from build123d import *

# Parameters (mm, degrees)
SKETCH1_W            = 34.7
SKETCH1_H            = 30
BOSS_EXTRUDE1_DEPTH  = 37.282
SKETCH4_R            = 5.715
CUT_EXTRUDE1_DEPTH   = 31
SKETCH8_W            = 3.81
SKETCH8_H            = 50.8
BOSS_EXTRUDE6_DEPTH  = 45.72
BOSS_EXTRUDE7_DEPTH  = 41.000001
CUT_EXTRUDE2_REACH   = 82.42
SKETCH10_R           = 1.905
SKETCH11_W           = 12.7
SKETCH11_H           = 44.810000611
BOSS_EXTRUDE8_DEPTH  = 12.7
SKETCH12_W           = 12.7
SKETCH12_H           = 44.810000611
BOSS_EXTRUDE9_DEPTH  = 12.7
SKETCH13_R           = 4.25
CUT_EXTRUDE3_DEPTH   = 6.35
SKETCH17_W           = 3.43592392
SKETCH17_H           = 45.72
BOSS_EXTRUDE12_DEPTH = 33.472
SKETCH16_W           = 2.5
SKETCH16_H           = 37.282
BOSS_EXTRUDE11_DEPTH = 9.076061
SKETCH21_W           = 17.974491303
SKETCH21_H           = 23.94
BOSS_EXTRUDE13_DEPTH = 16
SKETCH22_W           = 13.379509134
SKETCH22_H           = 6.922502695
CUT_EXTRUDE4_DEPTH   = 45.810000611
SKETCH23_W           = 13.335762063
SKETCH23_H           = 11.735762062
CUT_EXTRUDE5_DEPTH   = 21.47692
SKETCH24_W           = 22.672584076
SKETCH24_H           = 14.765845737
BOSS_EXTRUDE14_DEPTH = 15
SKETCH25_W           = 12.9
SKETCH25_H           = 11.3
CUT_EXTRUDE6_DEPTH   = 22.672584
SKETCH5_R            = 1.375
CUT_EXTRUDE7_DEPTH   = 10
SKETCH6_R            = 1.27
CUT_EXTRUDE8_DEPTH   = 53.282
SKETCH27_W           = 17.974491303
SKETCH27_H           = 14.491353785
BOSS_EXTRUDE15_DEPTH = 2


with BuildPart() as part:
    # Sketch1 → Boss-Extrude1 (new body)
    with BuildSketch(Plane(origin=(0, 0, -264.675), x_dir=(-1, 0, 0), z_dir=(0, 0, -1))):
        with Locations((-46.026450848, -396.896376681)):
            Rectangle(SKETCH1_W, SKETCH1_H)
    extrude(amount=BOSS_EXTRUDE1_DEPTH)

    # Sketch4 → Cut-Extrude1 (cut, through all)
    with BuildSketch(Plane(origin=(0, -381.896376681, 0), x_dir=(1, 0, 0), z_dir=(0, 1, 0))):
        with Locations((46.026450848, 283.749893694)):
            Circle(SKETCH4_R)
    extrude(amount=-CUT_EXTRUDE1_DEPTH, mode=Mode.SUBTRACT)

    # Sketch8 → Boss-Extrude6 (add)
    with BuildSketch(Plane(origin=(63.376450848, 0, 0), x_dir=(0, 0, -1), z_dir=(1, 0, 0))):
        with Locations((266.58, -395.572437442)):
            Rectangle(SKETCH8_W, SKETCH8_H)
    extrude(amount=BOSS_EXTRUDE6_DEPTH)

    # Sketch9 → Boss-Extrude7 (add)
    with BuildSketch(Plane(origin=(0, 0, -268.485), x_dir=(-1, 0, 0), z_dir=(0, 0, -1))):
        Polygon((-109.096450848, -370.172437442), (-63.376450848, -370.172437442), (-63.376450848, -372.712437442), (-106.556450848, -372.712437442), (-106.556450848, -384.142437442), (-109.096450848, -384.142437442), (-109.096450848, -372.712437442), align=None)
        Polygon((-109.096450848, -420.972437442), (-63.376450848, -420.972437442), (-63.376450848, -418.432437442), (-106.556450848, -418.432437442), (-106.556450848, -407.002437442), (-109.096450848, -407.002437442), (-109.096450848, -418.432437442), align=None)
    extrude(amount=BOSS_EXTRUDE7_DEPTH)

    # Sketch10 → Cut-Extrude2 (cut, up to next)
    with BuildSketch(Plane(origin=(109.096450848, 0, 0), x_dir=(0, 0, -1), z_dir=(1, 0, 0)), mode=Mode.PRIVATE) as cut_extrude2_sk1:
        with Locations((304.963451053, -379.773986799)):
            Circle(SKETCH10_R)
    cut_extrude2_tool1 = extrude(cut_extrude2_sk1.sketch, amount=-CUT_EXTRUDE2_REACH, mode=Mode.PRIVATE) & part.part
    add(cut_extrude2_tool1.solids().sort_by_distance((109.096451, -379.773987, -304.963451))[0], mode=Mode.SUBTRACT)
    # Sketch10 → Cut-Extrude2 (cut, up to next)
    with BuildSketch(Plane(origin=(109.096450848, 0, 0), x_dir=(0, 0, -1), z_dir=(1, 0, 0)), mode=Mode.PRIVATE) as cut_extrude2_sk2:
        with Locations((304.941901697, -411.752437852)):
            Circle(SKETCH10_R)
    cut_extrude2_tool2 = extrude(cut_extrude2_sk2.sketch, amount=-CUT_EXTRUDE2_REACH, mode=Mode.PRIVATE) & part.part
    add(cut_extrude2_tool2.solids().sort_by_distance((109.096451, -411.752438, -304.941902))[0], mode=Mode.SUBTRACT)
    # Sketch10 → Cut-Extrude2 (cut, up to next)
    with BuildSketch(Plane(origin=(109.096450848, 0, 0), x_dir=(0, 0, -1), z_dir=(1, 0, 0)), mode=Mode.PRIVATE) as cut_extrude2_sk3:
        with Locations((273.239000003, -379.752437442)):
            Circle(SKETCH10_R)
    cut_extrude2_tool3 = extrude(cut_extrude2_sk3.sketch, amount=-CUT_EXTRUDE2_REACH, mode=Mode.PRIVATE) & part.part
    add(cut_extrude2_tool3.solids().sort_by_distance((109.096451, -379.752437, -273.239))[0], mode=Mode.SUBTRACT)
    # Sketch10 → Cut-Extrude2 (cut, up to next)
    with BuildSketch(Plane(origin=(109.096450848, 0, 0), x_dir=(0, 0, -1), z_dir=(1, 0, 0)), mode=Mode.PRIVATE) as cut_extrude2_sk4:
        with Locations((273.221901697, -411.730888495)):
            Circle(SKETCH10_R)
    cut_extrude2_tool4 = extrude(cut_extrude2_sk4.sketch, amount=-CUT_EXTRUDE2_REACH, mode=Mode.PRIVATE) & part.part
    add(cut_extrude2_tool4.solids().sort_by_distance((109.096451, -411.730888, -273.221902))[0], mode=Mode.SUBTRACT)

    # Sketch11 → Boss-Extrude8 (add)
    with BuildSketch(Plane(origin=(0, -370.172437442, 0), x_dir=(1, 0, 0), z_dir=(0, 1, 0))):
        with Locations((102.746450848, 287.080000305)):
            Rectangle(SKETCH11_W, SKETCH11_H)
    extrude(amount=BOSS_EXTRUDE8_DEPTH)

    # Sketch12 → Boss-Extrude9 (add)
    with BuildSketch(Plane.XZ.offset(420.972437442)):
        with Locations((102.746450848, -287.080000305)):
            Rectangle(SKETCH12_W, SKETCH12_H)
    extrude(amount=BOSS_EXTRUDE9_DEPTH)

    # Sketch13 → Cut-Extrude3 (cut)
    with BuildSketch(Plane(origin=(109.096450848, 0, 0), x_dir=(0, 0, -1), z_dir=(1, 0, 0))):
        with Locations((288.985000522, -366.472437442)):
            Circle(SKETCH13_R)
        with Locations((288.985000522, -425.654437442)):
            Circle(SKETCH13_R)
    extrude(amount=-CUT_EXTRUDE3_DEPTH, mode=Mode.SUBTRACT)

    # Sketch17 → Boss-Extrude12 (add)
    with BuildSketch(Plane(origin=(0, 0, -268.485), x_dir=(-1, 0, 0), z_dir=(0, 0, -1))):
        with Locations((-65.094412808, -395.572437442)):
            Rectangle(SKETCH17_W, SKETCH17_H)
    extrude(amount=BOSS_EXTRUDE12_DEPTH)

    # Sketch16 → Boss-Extrude11 (add)
    with BuildSketch(Plane.XZ.offset(411.896376681)):
        with Locations((62.126450848, -283.316)):
            Rectangle(SKETCH16_W, SKETCH16_H)
    extrude(amount=BOSS_EXTRUDE11_DEPTH)

    # Sketch21 → Boss-Extrude13 (add)
    with BuildSketch(Plane(origin=(0, 0, -309.485000611), x_dir=(-1, 0, 0), z_dir=(0, 0, -1))):
        with Locations((-67.875046239, -432.942437442)):
            Rectangle(SKETCH21_W, SKETCH21_H)
    extrude(amount=-BOSS_EXTRUDE13_DEPTH)

    # Sketch22 → Cut-Extrude4 (cut, through all)
    with BuildSketch(Plane(origin=(0, 0, -309.485000611), x_dir=(-1, 0, 0), z_dir=(0, 0, -1))):
        with Locations((-67.562480009, -426.896769229)):
            Rectangle(SKETCH22_W, SKETCH22_H)
    extrude(amount=-CUT_EXTRUDE4_DEPTH, mode=Mode.SUBTRACT)

    # Sketch23 → Cut-Extrude5 (cut)
    with BuildSketch(Plane.XZ.offset(444.912437442)):
        with Locations((67.776450849, -303.385000611)):
            Rectangle(SKETCH23_W, SKETCH23_H)
    extrude(amount=-CUT_EXTRUDE5_DEPTH, mode=Mode.SUBTRACT)

    # Sketch24 → Boss-Extrude14 (add)
    with BuildSketch(Plane.XY.offset(-264.675)):
        with Locations((97.76015881, -394.484447642)):
            Rectangle(SKETCH24_W, SKETCH24_H)
    extrude(amount=BOSS_EXTRUDE14_DEPTH)

    # Sketch25 → Cut-Extrude6 (cut)
    with BuildSketch(Plane(origin=(109.096450848, 0, 0), x_dir=(0, 0, -1), z_dir=(1, 0, 0))):
        with Locations((257.775, -394.422437442)):
            Rectangle(SKETCH25_W, SKETCH25_H)
    extrude(amount=-CUT_EXTRUDE6_DEPTH, mode=Mode.SUBTRACT)

    # Sketch5 → Cut-Extrude7 (cut)
    with BuildSketch(Plane.XZ.offset(411.896376681)):
        with Locations((46.453266338, -275.535975412)):
            Circle(SKETCH5_R)
        with Locations((54.24036913, -284.176709184)):
            Circle(SKETCH5_R)
        with Locations((45.599635358, -291.963811975)):
            Circle(SKETCH5_R)
        with Locations((37.812532567, -283.323078204)):
            Circle(SKETCH5_R)
    extrude(amount=-CUT_EXTRUDE7_DEPTH, mode=Mode.SUBTRACT)

    # Sketch6 → Cut-Extrude8 (cut, through all)
    with BuildSketch(Plane(origin=(0, 0, -301.957), x_dir=(-1, 0, 0), z_dir=(0, 0, -1))):
        with Locations((-58.776450848, -387.896376681)):
            Circle(SKETCH6_R)
        with Locations((-33.276450848, -387.896376681)):
            Circle(SKETCH6_R)
        with Locations((-33.276450848, -405.896376681)):
            Circle(SKETCH6_R)
        with Locations((-58.776450848, -405.896376681)):
            Circle(SKETCH6_R)
    extrude(amount=-CUT_EXTRUDE8_DEPTH, mode=Mode.SUBTRACT)

    # Sketch27 → Boss-Extrude15 (add)
    with BuildSketch(Plane(origin=(0, 0, -309.485000611), x_dir=(-1, 0, 0), z_dir=(0, 0, -1))):
        with Locations((-67.875046239, -437.66676055)):
            Rectangle(SKETCH27_W, SKETCH27_H)
    extrude(amount=BOSS_EXTRUDE15_DEPTH)


solid = part.part
Could you check a few things on this model? Use its own coordinates, in mm. A direction names the side the tool comes from. Give positions to 0.01 mm unless a question says otherwise; leave off trailing zeros. Loops run counter-clockwise (first coordinate to the right, second up) from the corner with the lowest first, then second, coordinate; pieces in that order, holes last. Notation, with made-up numbers: (-33, -5) -> (17, -5) arc R30 ccw to (17, 18) -> close; hole circle Ø11 at (43.5, -16). An arc over 180 degrees is marked (long way). Answer as CSV lines item,"result". Start each with the question number.
(1) We'd pull the mould along Z, two halves only. Please class faces 1 (the flat face through (98, -395, -264.225)), 2 (the flat face through (81, -370.172, -287)), 3 (the flat face through (90, -372, -309.485)): released by +Z, released by -Z, zero draft, split by the parting line, or undercut.
(2) If we section it at D-D on z = -280: Write out the boundary of the cut face in (x, y), then the cut area to 3 significant figures.
(3) I need wall thicknesses on probe 1 along X at (y, z) = (-431.5, -302); probe 2 along Y at (x, z) = (73, -271); probe 3 along Y at (x, z) = (34, -295). Which ranges of each line are inside material? Lowest first, please.
(4) I'm going to push flat-ended pins straight in: pin 1 Ø18.5 at (x, z) = (46.03, -283.75) entering from -Y; pin 2 Ø20 at (x, y) = (67.5, -427.5) entering from +Z (3 decimals); pin 3 Ø10 at (x, y) = (77.5, -413.5) entering from -Z (3 decimals); pin 4 Ø10.5 at (x, y) = (70.5, -426) entering from -Z (3 decimals). Where does each tip first touch, or does it pass through?
(5) Which directions (+Z, -Z, +X, -X, +Y, -Y) give clear straight access to the entire face, cutting with the end or side of a thin tool? Please do faces 4 (the cylindrical face through (44.51, -406.97, -292.8)), 5 (the flat face through (98, -388.772, -258)), 6 (the flat face through (61, -420.972, -303)).
(6) If we section it at A-A on x = 72: Write out the boundary of the cut face in (y, z) (3 decimals), then the cut area to 3 significant figures.
(7) If we section it at B-B on y = -395.5: Write out the boundary of the cut face in (x, z) (3 decimals), then the cut area to 3 significant figures.
(8) If we section it at C-C on z = -255.5: Write out the boundary of the cut face in (x, y), then the cut area to 3 significant figures.
Computed:
1,face 1,"undercut"
1,face 2,"zero draft"
1,face 3,"released by -Z"
2,outline,"(28.68, -411.9) -> (41.71, -411.9) -> (41.71, -381.9) -> (28.68, -381.9) -> close; (50.34, -411.9) -> (60.88, -411.9) -> (60.88, -420.97) -> (96.4, -420.97) -> (96.4, -433.67) -> (109.1, -433.67) -> (109.1, -407) -> (106.56, -407) -> (106.56, -418.43) -> (66.81, -418.43) -> (66.81, -372.71) -> (106.56, -372.71) -> (106.56, -384.14) -> (109.1, -384.14) -> (109.1, -357.47) -> (96.4, -357.47) -> (96.4, -370.17) -> (63.38, -370.17) -> (63.38, -381.9) -> (50.34, -381.9) -> close; hole circle Ø2.54 at (33.28, -405.9); hole circle Ø2.54 at (33.28, -387.9); hole circle Ø2.54 at (58.78, -405.9); hole circle Ø2.54 at (58.78, -387.9)"
2,area,"1,550 mm2"
3,probe 1,"x = 58.89 to 61.11, 74.44 to 76.86, 96.4 to 109.1"
3,probe 2,"y = -420.97 to -418.43, -372.71 to -370.17"
3,probe 3,"y = -411.9 to -406.94, -404.85 to -388.94, -386.85 to -381.9"
4,pin 1,"stops at y = -411.9"
4,pin 2,"stops at z = -264.675"
4,pin 3,"stops at z = -309.485"
4,pin 4,"stops at z = -311.485"
5,face 4,"-Y"
5,face 5,"+X, -X"
5,face 6,"-Z, -X"
6,outline,"(-444.912, -311.485) -> (-430.421, -311.485) -> (-430.421, -309.485) -> (-430.358, -309.485) -> (-430.358, -309.253) -> (-444.912, -309.253) -> close; (-444.912, -297.517) -> (-430.358, -297.517) -> (-430.358, -293.485) -> (-444.912, -293.485) -> close; (-423.436, -309.485) -> (-418.432, -309.485) -> (-418.432, -268.485) -> (-372.712, -268.485) -> (-372.712, -309.485) -> (-370.172, -309.485) -> (-370.172, -264.675) -> (-420.972, -264.675) -> (-420.972, -293.485) -> (-423.436, -293.485) -> close"
6,area,"532 mm2"
7,outline,"(28.676, -301.957) -> (66.812, -301.957) -> (66.812, -268.485) -> (109.096, -268.485) -> (109.096, -264.225) -> (86.424, -264.225) -> (86.424, -264.675) -> (28.676, -264.675) -> close; (86.424, -251.325) -> (109.096, -251.325) -> (109.096, -249.675) -> (86.424, -249.675) -> close; hole circle Ø11.43 at (46.026, -283.75)"
7,area,"1,530 mm2"
8,outline,"(86.42, -401.87) -> (109.1, -401.87) -> (109.1, -400.07) -> (86.42, -400.07) -> close; (86.42, -388.77) -> (109.1, -388.77) -> (109.1, -387.1) -> (86.42, -387.1) -> close"
8,area,"78.6 mm2"
